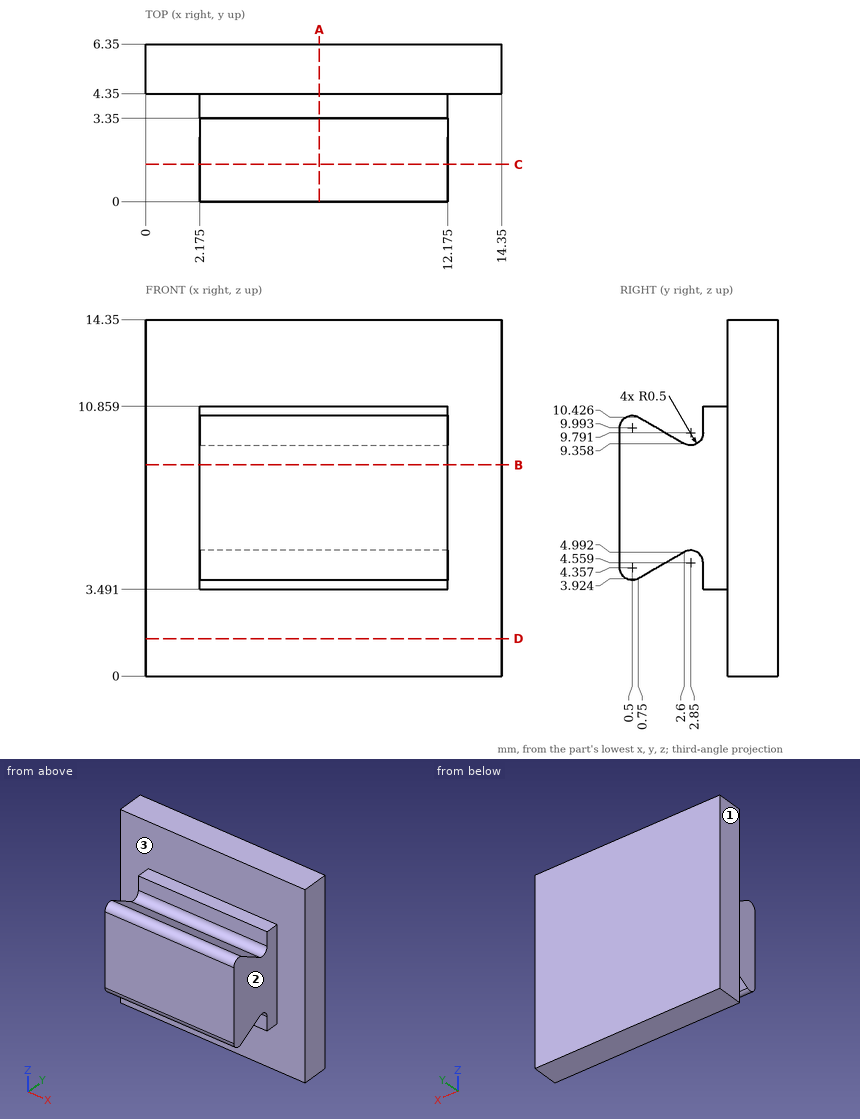
Answer from the drawing. Dimensions are ordinates in mm from the lowest x, y and z of the part. Give positions to 0.01 mm unless a question says otherwise; leave off trailing zeros. Loops run counter-clockwise (first coordinate to the right, second up) from the corner with the lowest first, then second, coordinate; pieces in that order, holes last. Notation, with made-up numbers: (75, 83) -> (123, 83) arc R20 cw to (123, 92) -> close; hole circle Ø2 at (83.25, 24). An arc over 180 degrees is marked (long way). Use a Markdown table: item, result.
Q1. Section D-D, the plane z = 1.5 is taken. Determine the outline of the cut face in (x, y).
Solved:
| item | result |
|---|---|
| outline | (0, 4.35) -> (14.35, 4.35) -> (14.35, 6.35) -> (0, 6.35) -> close |
Q2. Section A-A, the plane x = 7 is taken. Determine the outline of the cut face in (y, z).
Solved:
| item | result |
|---|---|
| outline | (0, 4.36) arc R0.5 ccw to (0.75, 3.92) -> (2.6, 4.99) arc R0.5 cw to (3.35, 4.56) -> (3.35, 3.49) -> (4.35, 3.49) -> (4.35, 0) -> (6.35, 0) -> (6.35, 14.35) -> (4.35, 14.35) -> (4.35, 10.86) -> (3.35, 10.86) -> (3.35, 9.79) arc R0.5 cw to (2.6, 9.36) -> (0.75, 10.43) arc R0.5 ccw to (0, 9.99) -> close |
Q3. Determine the mould class of the marked faces 1, 2 and 3 for opening direction X: pulls with the +X half, pulls with the -X half, needs draft (parallel to the pull), parting line crosses it, or undercut.
Solved:
| item | result |
|---|---|
| face 1 | pulls with the -X half |
| face 2 | pulls with the +X half |
| face 3 | needs draft |
Q4. Each of these flat-tipped pins is pushed along its axis until it touches: pin 1 (2 mm diameter, centred on y = 2, z = 7, fed in from -X) (3 decimals); pin 2 (2 mm diameter, centred on y = 2, z = 7.5, fed in from +X) (3 decimals); pin 3 (1.2 mm diameter, centred on x = 6.5, z = 10.5, fed in from -Y); pin 4 (1.5 mm diameter, centred on x = 9.5, y = 3.5, fed in from +Z). Where does it stop, or does it pass through?
Solved:
| item | result |
|---|---|
| pin 1 | stops at x = 2.175 |
| pin 2 | stops at x = 12.175 |
| pin 3 | stops at y = 0 |
| pin 4 | stops at z = 10.86 |
Q5. Find the intervals of material crossed by line 1 along Y through (x, z) = (2, 5); line 2 along X through (y, z) = (2.5, 6) (3 decimals); line 3 along Z through (x, y) = (4.5, 1.5), in increasing order.
Solved:
| item | result |
|---|---|
| line 1 | y = 4.35 to 6.35 |
| line 2 | x = 2.175 to 12.175 |
| line 3 | z = 4.36 to 9.99 |
Q6. Section B-B, the plane z = 8.5 is taken. Determine the outline of the cut face in (x, y) (3 decimals).
Solved:
| item | result |
|---|---|
| outline | (0, 4.35) -> (2.175, 4.35) -> (2.175, 0) -> (12.175, 0) -> (12.175, 4.35) -> (14.35, 4.35) -> (14.35, 6.35) -> (0, 6.35) -> close |
Q7. Section C-C, the plane y = 1.5 is taken. Determine the outline of the cut face in (x, z) (3 decimals), then the cut area to 3 significant figures.
Solved:
| item | result |
|---|---|
| outline | (2.175, 4.357) -> (12.175, 4.357) -> (12.175, 9.993) -> (2.175, 9.993) -> close |
| area | 56.4 mm^2 |
